Geometry: final body of the model. Coordinates: model frame, mm. A direction names the side the tool comes from. Give positions to 0.01 mm unless a question says otherwise; leave off trailing zeros. Use CSV: the item, a comma, the result in double quotes.
Autodesk Inventor part; units mm, degrees
ref_plane "Work Plane1" through (29, 0, 0) normal (0, -1, 0) x (1, 0, 0)
ref_plane "YZ Plane" through (0, 0, 0) normal (1, 0, 0) x (0, 1, 0)
ref_plane "XZ Plane" through (0, 0, 0) normal (0, 1, 0) x (-1, 0, 0)
sketch "Skizze1" plane through (0, 0, 0) normal (0, 0, 1) x (1, 0, 0)
  line L0 (-1, 0) -> (30, 0)
  line L1 (30, 0) -> (30, 2)
  line L2 (30, 2) -> (10, 2)
  line L3 (10, 2) -> (9.5705, 2)
  line L4 (9.5705, 2) -> (0, 2)
  line L5 (0, 2) -> (0, 3.5)
  line L6 (0, 3.5) -> (-4, 3.5)
  line L7 (-4, 3.5) -> (-4, 1.7321)
  line L8 (-4, 1.7321) -> (-2, 1.7321)
  line L9 (-2, 1.7321) -> (-1, 0)
  line L10 (-10.8, 0) -> (36.8, 0)
  line L11 (0, -0.7) -> (0, 4.2)
  line L12 (10, 2) -> (0, 2) construction
  dimension "d1" = 20
  dimension "d2" = 0.4295
  dimension "d3" = 4
  dimension "d4" = 2
  dimension "d5" = 60
  dimension "d6" = 4
  dimension "d7" = 4
  dimension "d8" = 3.4641
  dimension "d9" = 7
  dimension "d26" = 30
revolve "Körper" add sketch "Skizze1" angle 360 about axis through (-1, 0, 0) along (1, 0, 0)
sketch "Skizze2" plane through (-4, 0, 0) normal (-1, 0, 0) x (0, 0, 1)
  circle A0 centre (0, 0) radius 1.7321
  line L0 (0, -4.9) -> (0, 4.9)
  line L1 (-4.9, 0) -> (4.9, 0)
  line L2 (1.7321, 0) -> (0.866, -1.5)
  line L3 (0.866, -1.5) -> (-0.866, -1.5)
  line L4 (-0.866, -1.5) -> (-1.7321, 0)
  line L5 (-1.7321, 0) -> (-0.866, 1.5)
  line L6 (-0.866, 1.5) -> (0.866, 1.5)
  line L7 (0.866, 1.5) -> (1.7321, 0)
extrude "Loch" add sketch "Skizze2" against normal up to next contours L7 A0 | A0 L2 | L6 L0 A0 | A0 L0 L3 | L0 L6 A0 | A0 L3 L0 | L4 A0 | A0 L5
fillet "Rundung1" radius 0.4 1 edges at (-4, -3.5, 0)
thread "Gewinde"
chamfer "Fase1" distance 0.4294 distance2 0.4294 1 edges at (30, -2, 0) measured on face at (30, 0.0262, -0.4421)
ref_plane "Work Plane1" through (29, 0, 0) normal (0, -1, 0) x (1, 0, 0)
fillet "Fillet2" radius 0.2 1 edges at (0, -2, 0)
equation "\"d1\" = GEL"
equation "\"d3\" = KOH"
equation "\"d4\" = INTI"
equation "\"d6\" = GD"
equation "\"d7\" = BDM"
equation "\"d8\" = 1.1547 * SW"
equation "\"d9\" = KOD"
equation "\"d26\" = NLG"
equation "\"d30\" = R"
equation "\"d17\" = RR"
equation "\"d13\" = GEL"
equation "\"d15\" = -0.5 * SPD + 0.5 * GD"
equation "\"d16\" = GUL"
equation "\"GD\" = NND"
equation "\"NLG\" = 30"
equation "\"GEL\" = 20"
equation "\"KOD\" = 7"
equation "\"KOH\" = 4"
equation "\"INTI\" = 2"
equation "\"GAL\" = 0.61345 * PTC"
equation "\"GUL\" = 0.61345 * PTC"
equation "\"BDM\" = NND"
equation "\"SW\" = 3"
equation "\"RR\" = 0.4"
equation "\"SPD\" = NND - 1.2269 * PTC"
equation "\"R\" = 0.2"
equation "\"TOA\" = 30deg"
equation "\"GD1\" = THREADDIA - 1.2269 * PTC"
equation "\"THREADDIA\" = 4"
equation "\"FAWI\" = 45deg"
equation "\"ANG\" = 120deg"
equation "\"PTC\" = 0.7"
equation "\"NND\" = 4"
equation "\"E0\" = 1.155 * SW"
properties part number "DIN 912 - M4 x 30" material "Stahl, weich"
1. Pin query (flat end, axial travel): pin 1 Ø2 at (x, z) = (21.5, -2) entering from +Y. Return the tip coordinate at first contact, or that it passes through.
Answer:
pin 1,"y = 1.73"
2. Pull-direction query (Z, two-part tool) for faces 4 (the face through (-1.825, 3.233, 1.341)), 5 (the face through (-1, 0, 0)), 6 (the face through (30, 0, 0)); classes: +Z half, -Z half, draft (parallel to the pull), parting line (faces both ways), or undercut.
Answer:
face 4,"parting line"
face 5,"undercut"
face 6,"draft"
3. Reachability of faces 1 (the face through (-2.948, -0.761, -1.293)), 2 (the face through (0, -2, -2)), 3 (the face through (-4, -1.3, 1.3)) from +Z, -Z, +X, -X, +Y, -Y: full face, straight path, thin tool, end or side. Return the list, or none.
Answer:
face 1,"-X"
face 2,"+X"
face 3,"+Z, -Z, -X, +Y, -Y"
4. Line query: line 1 (X direction, y = -2.5, z = -1.5); line 2 (Z direction, x = 22.5, y = -1); line 3 (Z direction, x = -2, y = 1). Output: solid intervals per line, ascending.
Answer:
line 1,"-4 to 0"
line 2,"-1.73 to 1.73"
line 3,"-3.35 to -1.15, 1.15 to 3.35"
